```python
from build123d import *

# Parameters (mm, degrees)
BOSS_EXTRUDE1_DEPTH             = 6.35
F_4_0MM_DOWEL_HOLE1_D           = 4
F_4_0MM_DOWEL_HOLE1_CSINK_D     = 4.05
F_4_0MM_DOWEL_HOLE1_CSINK_ANGLE = 90


with BuildPart() as part:
    # Sketch1 → Boss-Extrude1 (new body)
    with BuildSketch(Plane.XY):
        with BuildLine():
            Line((0, 0), (-8.732389132, 0))
            ThreePointArc((-8.732389132, 0), (-10.716194566, 1.746), (-12.7, 0))
            Line((-12.7, 0), (-12.7, 7.62))
            Line((-12.7, 7.62), (0, 7.62))
            Line((0, 7.62), (0, 0))
        make_face()
    extrude(amount=BOSS_EXTRUDE1_DEPTH)

    # Ø4.0mm Dowel Hole1 (through all)
    with Locations(Plane(origin=(0, 0, 0), x_dir=(-1, 0, 0), z_dir=(0, -1, 0))):
        with Locations((3.175, -3.175)):
            CounterSinkHole(F_4_0MM_DOWEL_HOLE1_D / 2, F_4_0MM_DOWEL_HOLE1_CSINK_D / 2, counter_sink_angle=F_4_0MM_DOWEL_HOLE1_CSINK_ANGLE)


solid = part.part
```
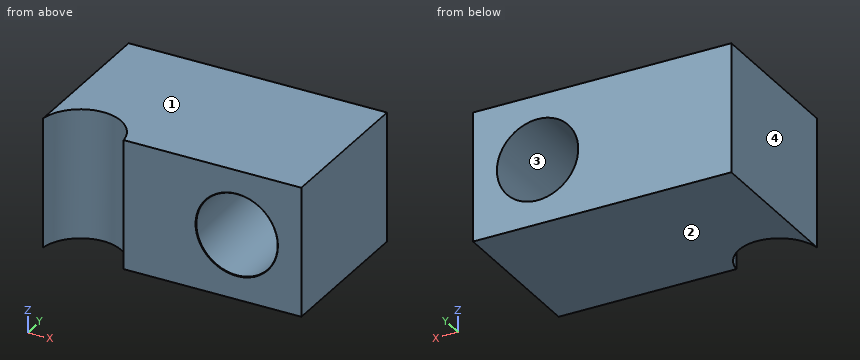
Source: CAD feature listing. Evaluate the final solid. Frame: model axes, mm. Face numbers are marked on the shaded views. Coordinates: 2 decimals unless noted, no trailing zeros. Write each loop counter-clockwise with the first axis right and the second up, starting at its lowest first coordinate (ties: lowest second). Pieces come first, ordered by that corner, then holes. Notation, with made-up numbers: (-18.75, 67) -> (-12.75, 67) arc R20 cw to (-12.75, 84) -> close; hole circle Ø3 at (26, 22). An arc over 180 degrees is marked (long way). Return JSON: item names as keys, results as strings. Group by question number.
1) Ray query, line 1 along X through (y, z) = (1.25, 4); line 2 along X through (y, z) = (1.5, 3.5); line 3 along Z through (x, y) = (-3, 4). Return the intervals inside material, ascending.
2) Section query B-B, the plane y = 3. Return loops of the section in (x, z) (3 decimals), plus the area to 3 significant figures.
3) Section query C-C, the plane x = -9.5. Return loops of the section in (y, z).
4) Mould query, pull axis Z, two halves, no side actions, for the marked faces 1, 2, 3 and 4. Classes: +Z half, -Z half, draft (parallel to the pull), parting line (faces both ways), or undercut.
5) Section query A-A, the plane z = 1. Return loops of the section in (x, y).
From the geometry:
{
 "1": {"line 1": "-12.7 to -12.03, -9.4 to -5, -1.35 to 0", "line 2": "-12.7 to -11.68, -9.76 to -5.15, -1.2 to 0", "line 3": "0 to 1.18, 5.17 to 6.35"},
 "2": {"outline": "(-12.7, 0) -> (0, 0) -> (0, 6.35) -> (-12.7, 6.35) -> close; hole circle Ø4 at (-3.175, 3.175)", "area": "68.1 mm²"},
 "3": {"outline": "(1.33, 0) -> (7.62, 0) -> (7.62, 6.35) -> (1.33, 6.35) -> close"},
 "4": {"face 1": "+Z half", "face 2": "-Z half", "face 3": "undercut", "face 4": "draft"},
 "5": {"outline": "(-12.7, 0) arc R2 cw to (-8.73, 0) -> (0, 0) -> (0, 7.62) -> (-12.7, 7.62) -> close"}
}
